The model under review builds one solid part; all positions refer to its coordinate system, in mm. Face numbers are marked on the shaded views. A direction names the side the tool comes from. Give positions to 0.01 mm unless a question says otherwise; leave off trailing zeros. Loops run counter-clockwise (first coordinate to the right, second up) from the corner with the lowest first, then second, coordinate; pieces in that order, holes last. Notation, with made-up numbers: M 80,52 L 85,52 A22 cw 85,74 Z; hole C -22,37 d7. An arc over 180 degrees is marked long. One line per item, written item: value. Start each with the question number.
Q1. For pin 1 (8 mm diameter, centred on x = -34, z = 65, fed in from -Y); pin 2 (6 mm diameter, centred on x = 75, z = 98, fed in from +Y); pin 3 (1 mm diameter, centred on x = -63.5, y = 37, fed in from +Z); pin 4 (8 mm diameter, centred on x = -43.5, y = 12.5, fed in from -Z), all flat-tipped, find the tip position at first contact; note any pin that passes through.
Q2. We need section B-B on y = 46. Give the number of separate pieces and of enclosed holes in the cut face, plus the area to 3 significant figures.
Q3. For the marked faces 4 and 5, list the 3-axis set-ups (+Z, -Z, +X, -X, +Y, -Y) from which the entire face can be reached by the end or side of a thin tool; tool diameter is ignored.
Q4. To check wall thickness, follow line 1 along Z through (x, y) = (0, 41); line 2 along X through (y, z) = (30, 6); line 3 along Y through (x, z) = (29, -99). State the ranges of each line that lie inside material, in increasing order. Write a range as from..to.
Q5. Mouldability with a two-part tool opening along X and no side actions: class the marked faces 1, 2 and 3 as released by +X, released by -X, zero draft, split by the parting line, or undercut.
Q6. We need section A-A on z = -61. Write out the cut boundary in (x, y), plus the area to 3 significant figures.
Q7. We need section C-C on z = -7. Write out the cut boundary in (x, y).
```python
from build123d import *

# Parameters (mm, degrees)
M5X0_8_TAPPED_HOLE1_D     = 4.2
M5X0_8_TAPPED_HOLE1_DEPTH = 17.399
M5X0_8_TAPPED_HOLE1_TIP   = 1.2618073
CUT_EXTRUDE1_REACH        = 188.651
SKETCH7_W                 = 50.8
SKETCH7_H                 = 2.565921067
CUT_EXTRUDE2_REACH        = 188.651
FILLET1_R                 = 1.5875
CIRPATTERN1_COUNT         = 9
FILLET1_OF_CIRPATTERN1_R  = 1.5875
SKETCH11_R                = 93
SKETCH11_R_2              = 89
CUT_EXTRUDE3_DEPTH        = 2


with BuildPart() as part:
    # Sketch1 → Revolve1 (revolve)
    with BuildSketch(Plane.XY):
        Polygon((80.3783, 0), (127, 0), (127, 6.35), (98.425, 6.35), (98.425, 20.32), (108, 20.32), (108, 50.8), (96.5, 50.8), (96.5, 31.3), (80.3783, 31.3), align=None)
    revolve(axis=Axis((0, 0, 0), (0, 1, 0)))

    # M5x0.8 Tapped Hole1
    with Locations(Plane(origin=(0, 50.8, 0), x_dir=(1, 0, 0), z_dir=(0, 1, 0))):
        with Locations((0, 102), (72.124891681, 72.124891681), (102, 0), (72.124891681, -72.124891681), (0, -102), (-72.124891681, -72.124891681), (-102, 0), (-72.124891681, 72.124891681)):
            Hole(M5X0_8_TAPPED_HOLE1_D / 2, depth=M5X0_8_TAPPED_HOLE1_DEPTH)
            with Locations((0, 0, -(M5X0_8_TAPPED_HOLE1_DEPTH + M5X0_8_TAPPED_HOLE1_TIP / 2))):  # 118° drill point
                Cone(0, M5X0_8_TAPPED_HOLE1_D / 2, M5X0_8_TAPPED_HOLE1_TIP, mode=Mode.SUBTRACT)

    # Sketch7 → Cut-Extrude1 (cut, up to next)
    with BuildSketch(Plane(origin=(0, 50.8, 0), x_dir=(1, 0, 0), z_dir=(0, 1, 0)), mode=Mode.PRIVATE) as cut_extrude1_sk1:
        with Locations((0, -125.717039467)):
            Rectangle(SKETCH7_W, SKETCH7_H)
    cut_extrude1_tool1 = extrude(cut_extrude1_sk1.sketch, amount=-CUT_EXTRUDE1_REACH, mode=Mode.PRIVATE) & part.part
    add(cut_extrude1_tool1.solids().sort_by_distance((0, 50.8, 125.717039))[0], mode=Mode.SUBTRACT)

    # Sketch10 → Cut-Extrude2 (cut, up to next)
    with BuildSketch(Plane.XZ, mode=Mode.PRIVATE) as cut_extrude2_sk1:
        with BuildLine():
            Line((-3.3782, -106.045), (-3.3782, -127))
            Line((-3.3782, -127), (3.3782, -127))
            Line((3.3782, -127), (3.3782, -106.045))
            ThreePointArc((3.3782, -106.045), (0, -102.6668), (-3.3782, -106.045))
        make_face()
    cut_extrude2_tool1 = extrude(cut_extrude2_sk1.sketch, amount=-CUT_EXTRUDE2_REACH, mode=Mode.PRIVATE) & part.part
    cut_extrude2 = cut_extrude2_tool1.solids().sort_by_distance((0, 0, -115.183843))[0]
    add(cut_extrude2, mode=Mode.SUBTRACT)

    # Fillet1
    fillet1_edges = [part.edges().sort_by_distance(p)[0] for p in [
        (-3.3782, 3.175, -126.95506199),
        (3.3782, 3.175, -126.95506199),
    ]]
    fillet(fillet1_edges, radius=FILLET1_R)

    # CirPattern1: Cut-Extrude2 ×9 about axis
    cirpattern1_axis = Axis((0, 0, 0), (0, 1, 0))
    for i in range(1, CIRPATTERN1_COUNT):
        add(cut_extrude2.rotate(cirpattern1_axis, i * 360 / CIRPATTERN1_COUNT), mode=Mode.SUBTRACT)

    # Fillet1 of CirPattern1
    fillet1_of_cirpattern1_edges = [part.edges().sort_by_distance(p)[0] for p in [
        (-84.192992172, 3.175, -95.08175466),
        (-79.017289496, 3.175, -99.424684866),
        (-125.612947605, 3.175, -18.718637609),
        (-124.439711058, 3.175, -25.372392711),
        (-108.257208822, 3.175, 66.403138014),
        (-111.635408822, 3.175, 60.551923976),
        (-40.246718886, 3.175, 120.454147371),
        (-46.595658109, 3.175, 118.143322475),
        (46.595658109, 3.175, 118.143322475),
        (40.246718886, 3.175, 120.454147371),
        (111.635408822, 3.175, 60.551923976),
        (108.257208822, 3.175, 66.403138014),
        (124.439711058, 3.175, -25.372392711),
        (125.612947605, 3.175, -18.718637609),
        (79.017289496, 3.175, -99.424684866),
        (84.192992172, 3.175, -95.08175466),
    ]]
    fillet(fillet1_of_cirpattern1_edges, radius=FILLET1_OF_CIRPATTERN1_R)

    # Sketch11 → Cut-Extrude3 (cut)
    with BuildSketch(Plane(origin=(0, 31.3, 0), x_dir=(1, 0, 0), z_dir=(0, 1, 0))):
        with Locations(Location((0, 0, 0), (0, 0, 180))):
            Circle(SKETCH11_R)
        with Locations(Location((0, 0, 0), (0, 0, 180))):
            Circle(SKETCH11_R_2, mode=Mode.SUBTRACT)
    extrude(amount=-CUT_EXTRUDE3_DEPTH, mode=Mode.SUBTRACT)


solid = part.part
```
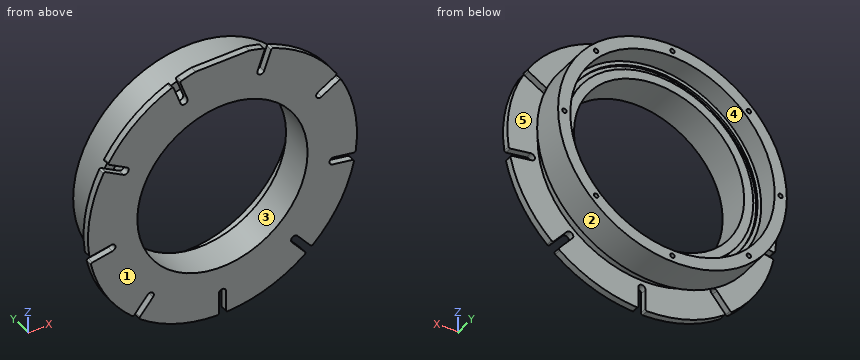
Solved:
1. pin 1: through
1. pin 2: y = 6.35
1. pin 3: z = 87.72
1. pin 4: z = -90.15
2. separate pieces: 1
2. enclosed holes: 9
2. area: 7,280 mm2
3. face 4: +Y
3. face 5: none
4. line 1: -108..-104.1, -99.9..-96.5, 96.5..99.9, 104.1..108
4. line 2: -107.83..-92.81, -88.8..-80.15, 80.15..88.8, 92.81..107.83
4. line 3: 0..6.35, 20.32..50.8
5. face 1: zero draft
5. face 2: split by the parting line
5. face 3: undercut
6. outline: M -111.39,0 L -52.34,0 L -52.34,31.3 L -64.81,31.3 L -64.81,29.3 L -70.2,29.3 L -70.2,31.3 L -74.77,31.3 L -74.77,50.8 L -89.12,50.8 L -89.12,20.32 L -77.24,20.32 L -77.24,6.35 L -111.39,6.35 Z; M 52.34,0 L 111.39,0 L 111.39,6.35 L 77.24,6.35 L 77.24,20.32 L 89.12,20.32 L 89.12,50.8 L 74.77,50.8 L 74.77,31.3 L 70.2,31.3 L 70.2,29.3 L 64.81,29.3 L 64.81,31.3 L 52.34,31.3 Z
6. area: 2,790 mm2
7. outline: M -126.81,0 L -80.07,0 L -80.07,31.3 L -88.72,31.3 L -88.72,29.3 L -92.74,29.3 L -92.74,31.3 L -96.25,31.3 L -96.25,50.8 L -107.77,50.8 L -107.77,20.32 L -98.18,20.32 L -98.18,6.35 L -126.81,6.35 Z; M 80.07,0 L 126.81,0 L 126.81,6.35 L 98.18,6.35 L 98.18,20.32 L 107.77,20.32 L 107.77,50.8 L 96.25,50.8 L 96.25,31.3 L 92.74,31.3 L 92.74,29.3 L 88.72,29.3 L 88.72,31.3 L 80.07,31.3 Z
